Verification items for this drawing (mm, ordinates from the low corner). A direction names the side the tool comes from. Coordinates: 2 decimals unless noted, no trailing zeros. Order: outer loops, then holes, each group sorted by start corner. A loop starts at its lowest first (then second) coordinate and runs counter-clockwise, first axis right, second up. Notation, with made-up numbers: (38.25, -27.5) -> (97.25, -27.5) arc R38 cw to (97.25, 10.5) -> close; hole circle Ø5 at (22.5, 10.25). An arc over 180 degrees is marked (long way). Answer in a Markdown table with one row per item. Add a question column.
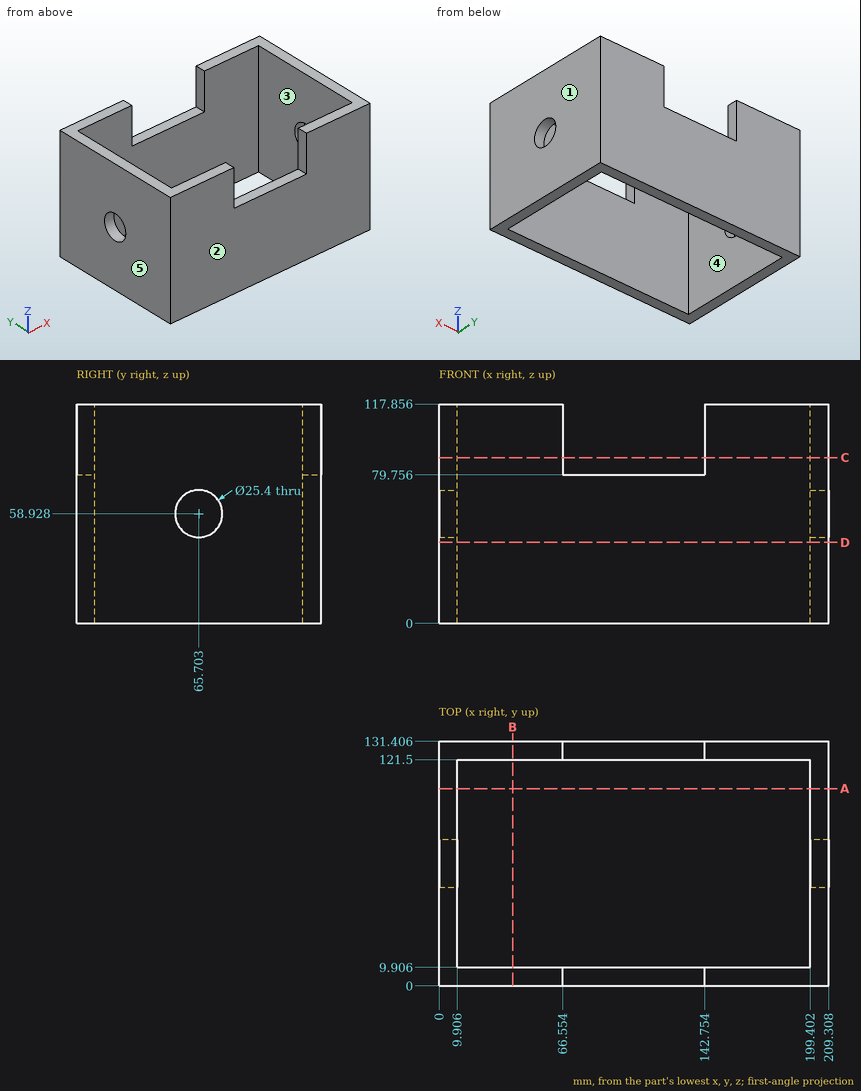
(1) Scan lines: line 1 along Y through (x, z) = (176, 107); line 2 along X through (y, z) = (61, 94); line 3 along Z through (x, y) = (132.5, 126.5). Record each from-to range of solid material in increasing order.
(2) Cross-section at A-A (y = 106). Enter the section's corners in (x, z).
(3) Cross-section at C-C (z = 89). Enter the section's corners in (x, y).
(4) Cross-section at B-B (x = 39.5). Enter the section's corners in (y, z), plus the area to 4 significant figures.
(5) Cross-section at D-D (z = 43.5). Enter the section's corners in (x, y).
(6) Go/stop test with flat-tipped pins: P1, Ø5, axis at y = 6.5, z = 103.5, coming from the -X side; P2, Ø3, axis at x = 89.5, y = 3, coming from the +Z side. Record where each tip stops, or that it passes through.
(7) Access from +Z, -Z, +X, -X, +Y, -Y to the whole of each face (thin tool, end or side, straight path). Record for the marked faces 4 and 5.
(8) Mould release check, pull along Y, two halves, no side actions. Record for the marked faces 1, 2 and 3: +Y half, -Y half, draft (parallel to the pull), parting line (faces both ways), or undercut.
Checks:
| question | item | result |
|---|---|---|
| 1 | line 1 | 0 to 9.91, 121.5 to 131.41 |
| 1 | line 2 | 0 to 9.91, 199.4 to 209.31 |
| 1 | line 3 | 0 to 79.76 |
| 2 | outline | (0, 0) -> (9.91, 0) -> (9.91, 117.86) -> (0, 117.86) -> close; (199.4, 0) -> (209.31, 0) -> (209.31, 117.86) -> (199.4, 117.86) -> close |
| 3 | outline | (0, 0) -> (66.55, 0) -> (66.55, 9.91) -> (9.91, 9.91) -> (9.91, 121.5) -> (66.55, 121.5) -> (66.55, 131.41) -> (0, 131.41) -> close; (142.75, 0) -> (209.31, 0) -> (209.31, 131.41) -> (142.75, 131.41) -> (142.75, 121.5) -> (199.4, 121.5) -> (199.4, 9.91) -> (142.75, 9.91) -> close |
| 4 | outline | (0, 0) -> (9.91, 0) -> (9.91, 117.86) -> (0, 117.86) -> close; (121.5, 0) -> (131.41, 0) -> (131.41, 117.86) -> (121.5, 117.86) -> close |
| 4 | area | 2,335 mm² |
| 5 | outline | (0, 0) -> (209.31, 0) -> (209.31, 131.41) -> (0, 131.41) -> close; hole (9.91, 9.91) -> (199.4, 9.91) -> (199.4, 121.5) -> (9.91, 121.5) -> close |
| 6 | P1 | x = 0 |
| 6 | P2 | z = 79.76 |
| 7 | face 4 | +Z, -Z |
| 7 | face 5 | +Z, -Z, -X, +Y, -Y |
| 8 | face 1 | draft |
| 8 | face 2 | -Y half |
| 8 | face 3 | undercut |
